```python
from build123d import *

# Parameters (mm, degrees)
SKETCH1_R                = 5
BOSS_EXTRUDE1_DEPTH      = 11
BOSS_EXTRUDE1_DEPTH_BACK = 3
SKETCH3_R                = 0.5
CUT_EXTRUDE1_DEPTH       = 11
CUT_EXTRUDE2_DEPTH       = 3


with BuildPart() as part:
    # Sketch1 → Boss-Extrude1 (new body, two sides)
    with BuildSketch(Plane.XY) as boss_extrude1_sk:
        Circle(SKETCH1_R)
        with BuildLine():
            Line((1.565247584, 2.2), (-1.565247584, 2.2))
            ThreePointArc((-1.565247584, 2.2), (0, -2.7), (1.565247584, 2.2))
        make_face(mode=Mode.SUBTRACT)
    extrude(amount=BOSS_EXTRUDE1_DEPTH)
    extrude(boss_extrude1_sk.sketch, amount=-BOSS_EXTRUDE1_DEPTH_BACK)

    # Sketch2 → Cut-Revolve1 (revolve, cut)
    with BuildSketch(Plane(origin=(0, 0, 0), x_dir=(0, 0, -1), z_dir=(1, 0, 0))):
        with BuildLine():
            Line((1, 5), (-1, 5))
            ThreePointArc((-1, 5), (0, 4), (1, 5))
        make_face()
    revolve(axis=Axis((0, 0, 0), (0, 0, 1)), mode=Mode.SUBTRACT)

    # Sketch3 → Cut-Extrude1 (cut)
    with BuildSketch(Plane(origin=(0, 0, 0), x_dir=(1, 0, 0), z_dir=(0, 1, 0))):
        Circle(SKETCH3_R)
    extrude(amount=CUT_EXTRUDE1_DEPTH, mode=Mode.SUBTRACT)

    # Sketch4 → Cut-Extrude2 (cut)
    with BuildSketch(Plane(origin=(0, 0, -3), x_dir=(-1, 0, 0), z_dir=(0, 0, -1))):
        with BuildLine():
            Line((-0.5, 2.2), (0.5, 2.2))
            ThreePointArc((0.5, 2.2), (0, 2.7), (-0.5, 2.2))
        make_face()
    extrude(amount=-CUT_EXTRUDE2_DEPTH, mode=Mode.SUBTRACT)


solid = part.part
```
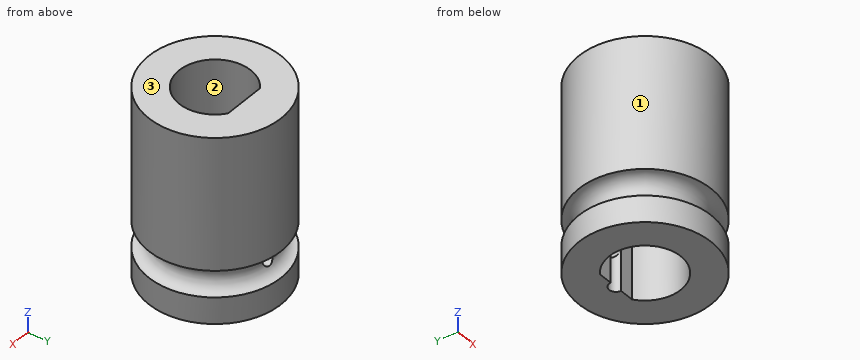
Input: part model. Units: mm. Frame: model coordinates. Face numbers are marked on the shaded views. Round coordinates to 2 decimals unless told otherwise and drop trailing zeros. Loops run counter-clockwise (first coordinate to the right, second up) from the corner with the lowest first, then second, coordinate; pieces in that order, holes last.
1) Section query B-B on y = 0. Return the cut outline in (x, z).
Ans:
outline: (-5, -3) - (-2.7, -3) - (-2.7, 11) - (-5, 11) - (-5, 1) arc R1 cw to (-5, -1) - close; (2.7, -3) - (5, -3) - (5, -1) arc R1 cw to (5, 1) - (5, 11) - (2.7, 11) - close
2) Section query A-A on x = 0. Return the cut outline in (y, z), plus the area to 3 significant figures.
Ans:
outline: (-5, -3) - (-2.7, -3) - (-2.7, 11) - (-5, 11) - (-5, 1) arc R1 cw to (-5, -1) - close; (2.2, 0.5) - (4.13, 0.5) arc R1 cw to (5, 1) - (5, 11) - (2.2, 11) - close; (2.7, -3) - (5, -3) - (5, -1) arc R1 cw to (4.13, -0.5) - (2.7, -0.5) - close
area: 65.2 mm2
3) Material intervals for line 1 (Y direction, x = 0, z = 2); line 2 (Z direction, x = 0, y = 4); line 3 (X direction, y = 0, z = 2), sorted ascending.
Ans:
line 1: y = -5 to -2.7, 2.2 to 5
line 2: z = -3 to -0.5, 0.5 to 11
line 3: x = -5 to -2.7, 2.7 to 5
4) Pull-direction query (X, two-part tool) for the marked faces 1, 2 and 3; classes: released by +X, released by -X, zero draft, split by the parting line, or undercut.
Ans:
face 1: split by the parting line
face 2: undercut
face 3: zero draft
5) Section query C-C on z = 9.75. Return the cut outline in (x, y), plus the area to 3 significant figures.
Ans:
outline: circle Ø10 at (0, 0); hole (-1.57, 2.2) arc R2.7 ccw (long way) to (1.57, 2.2) - close
area: 56.7 mm2
6) Pin query (flat end, axial travel): pin 1 (1 mm diameter, centred on x = -1, y = 0.5, fed in from +Z). Return the tip coordinate at first contact, or that it passes through.
Ans:
pin 1: passes through
